from build123d import *

# Parameters (mm, degrees)
PAD002_DEPTH = 50
SKETCH005_R  = 1.25
POCKET_DEPTH = 20
FILLET_R     = 2
FILLET001_R  = 2


with BuildPart() as part:
    # Sketch002 → Pad002 (new body)
    with BuildSketch(Plane.YZ):
        with BuildLine():
            Line((0, 0), (10, 0))
            Line((10, 0), (10, 10))
            Line((10, 10), (29, 28))
            Line((29, 28), (5, 28))
            ThreePointArc((5, 28), (1.464466, 26.535534), (0, 23))
            Line((0, 23), (0, 0))
        make_face()
    extrude(amount=PAD002_DEPTH)

    # Sketch005 → Pocket (cut)
    with BuildSketch(Plane.XY):
        with Locations((5, 4)):
            Circle(SKETCH005_R)
        with Locations((15, 4)):
            Circle(SKETCH005_R)
        with Locations((25, 4)):
            Circle(SKETCH005_R)
        with Locations((35, 4)):
            Circle(SKETCH005_R)
        with Locations((45, 4)):
            Circle(SKETCH005_R)
    extrude(amount=POCKET_DEPTH, mode=Mode.SUBTRACT)

    # Fillet
    fillet_edges = [part.edges().sort_by_distance(p)[0] for p in [
        (25, 29, 28),
    ]]
    fillet(fillet_edges, radius=FILLET_R)

    # Fillet001
    fillet001_edges = [part.edges().sort_by_distance(p)[0] for p in [
        (50, 17.678161, 17.274047),
        (50, 25.838763, 26.740334),
        (50, 10, 5),
        (50, 14.490416, 28),
        (50, 5, 0),
        (50, 1.464466, 26.535534),
        (50, 0, 11.5),
        (0, 17.678161, 17.274047),
        (0, 25.838763, 26.740334),
        (0, 10, 5),
        (0, 14.490416, 28),
        (0, 5, 0),
        (0, 1.464466, 26.535534),
        (0, 0, 11.5),
    ]]
    fillet(fillet001_edges, radius=FILLET001_R)


with BuildPart() as part_1:
    # Body002 placement: moved
    add(part.part.moved(Location((0, 0, 4))))


solid = part_1.part
Work out the finished part from the listing and answer in its coordinate system (mm). A direction names the side the tool comes from. Give positions to 0.01 mm unless a question says otherwise; leave off trailing zeros. Write each loop counter-clockwise with the first axis right and the second up, starting at its lowest first coordinate (ties: lowest second). Pieces come first, ordered by that corner, then holes. Notation, with made-up numbers: (-9.75, 66.5) - (15.25, 66.5) arc R18 ccw to (15.25, 100.5) - close; hole circle Ø6 at (-24, 50). An arc over 180 degrees is marked (long way). One line per item, written item: value. Start each with the question number.
1. Find section B-B (x = 29.5). Write down the section's boundary in (y, z).
2. Consider probe 1 along Y at (x, z) = (5, 10); probe 2 along Y at (x, z) = (29, 11.5); probe 3 along Y at (x, z) = (15, 18.5). Determine where each line is inside the solid, lowest interval first.
3. For faces 5 (the flat face through (35, 4, 24)), 6 (the flat face through (25, 15, 32)), 7 (the flat face through (25, 10, 9)), determine the directions among +Z, -Z, +X, -X, +Y, -Y from which every point of the face is accessible in a straight line to the end or side of a thin tool.
4. Given pin 1 (8 mm diameter, centred on x = 17.5, z = 9.5, fed in from +Y); pin 2 (0.8 mm diameter, centred on x = 34.5, y = 4, fed in from -Z); pin 3 (10 mm diameter, centred on x = 40, z = 14.5, fed in from +Y), each flat-ended and moving along its own axis, determine where each tip first touches the part or whether it passes through.
5. Find section C-C (x = 15). Write down the section's boundary in (y, z).
6. For a pull along X with two mould halves and no side action, classify faces 1 (the flat face through (0, 8, 21)), 2 (the flat face through (5, 4, 24)), 3 (the cylindrical face through (26.155, 3.521, 13.86)), 4 (the cylindrical face through (49.4, 14.36, 31.43)) as +X half, -X half, draft (parallel to the pull), parting line (faces both ways), or undercut.
7. Find section D-D (z = 19). State how many separate pieces and enclosed holes the cut face has, then the cut area to 3 significant figures.
8. Find section A-A (z = 9.5). Write down the section's boundary in (x, y), then the cut area to 3 significant figures.
Geometry results:
1. outline: (0, 4) - (10, 4) - (10, 14) - (25.36, 28.55) arc R2 ccw to (23.98, 32) - (5, 32) arc R5 ccw to (0, 27) - close
2. probe 1: 0 to 2.75, 5.25 to 10
2. probe 2: 0 to 10
2. probe 3: 0 to 2.75, 5.25 to 14.75
3. face 5: -Z
3. face 6: +Z, +X, -X, +Y, -Y
3. face 7: -Z, +X, -X, +Y
4. pin 1: y = 10
4. pin 2: z = 24
4. pin 3: y = 15.81
5. outline: (0, 4) - (2.75, 4) - (2.75, 24) - (5.25, 24) - (5.25, 4) - (10, 4) - (10, 14) - (25.36, 28.55) arc R2 ccw to (23.98, 32) - (5, 32) arc R5 ccw to (0, 27) - close
6. face 1: -X half
6. face 2: undercut
6. face 3: undercut
6. face 4: +X half
7. separate pieces: 1
7. enclosed holes: 5
7. area: 735 mm2
8. outline: (0, 2) arc R2 ccw to (2, 0) - (48, 0) arc R2 ccw to (50, 2) - (50, 8) arc R2 ccw to (48, 10) - (2, 10) arc R2 ccw to (0, 8) - close; hole circle Ø2.5 at (5, 4); hole circle Ø2.5 at (15, 4); hole circle Ø2.5 at (25, 4); hole circle Ø2.5 at (35, 4); hole circle Ø2.5 at (45, 4)
8. area: 472 mm2
